The listing builds one solid part. Answer for the finished solid, in the listing's coordinates (mm). A direction names the side the tool comes from. Coordinates: 2 decimals unless noted, no trailing zeros. Order: outer loops, then holes, each group sorted by start corner. A loop starts at its lowest first (then second) coordinate and runs counter-clockwise, first axis right, second up. Notation, with made-up numbers: (9, 36) -> (33, 36) arc R19 ccw to (33, 49) -> close; hole circle Ø11 at (-10.75, 80). An arc over 180 degrees is marked (long way). Put each result on its own line as item: value. Start each with the question number.
```python
from build123d import *

# Parameters (mm, degrees)
SKETCH3_W               = 44.4
SKETCH3_H               = 44.4
BOSS_EXTRUDE1_DEPTH     = 9.7
SKETCH4_W               = 10.3
SKETCH4_H               = 10.3
CUT_EXTRUDE1_DEPTH      = 5.3
SKETCH5_R               = 6
CUT_EXTRUDE2_DEPTH      = 14.3
BOSS_EXTRUDE2_DEPTH     = 5
CUT_EXTRUDE3_DEPTH      = 35.870626966
CUT_EXTRUDE3_DEPTH_BACK = 35.870626966
SKETCH7_R               = 1.5


with BuildPart() as part:
    # Sketch2 → Revolve1 (revolve)
    with BuildSketch(Plane.XY, mode=Mode.PRIVATE) as revolve1_sk:
        with BuildLine():
            Line((-10, 0), (-12, 0))
            ThreePointArc((-12, 0), (-8.485281374, 8.485281374), (0, 12))
            Line((0, 12), (0, 17))
            ThreePointArc((0, 17), (-12.02081528, 12.02081528), (-17, 0))
            Line((-17, 0), (-17, -3.175))
            Line((-17, -3.175), (-10, -3.175))
            Line((-10, -3.175), (-10, 0))
        make_face()
    revolve(revolve1_sk.sketch.rotate(Axis((0, 12, 0), (0, 1, 0)), 180), axis=Axis((0, 12, 0), (0, 1, 0)))

    # Sketch3 → Boss-Extrude1 (add)
    with BuildSketch(Plane.XZ.offset(3.175)):
        Rectangle(SKETCH3_W, SKETCH3_H)
    extrude(amount=BOSS_EXTRUDE1_DEPTH)

    # Sketch4 → Cut-Extrude1 (cut)
    with BuildSketch(Plane.XZ.offset(12.875)):
        with Locations((17.05, -17.05)):
            Rectangle(SKETCH4_W, SKETCH4_H)
    extrude(amount=-CUT_EXTRUDE1_DEPTH, mode=Mode.SUBTRACT)

    # Sketch5 → Cut-Extrude2 (cut)
    with BuildSketch(Plane.XZ.offset(12.875)):
        Circle(SKETCH5_R)
    extrude(amount=-CUT_EXTRUDE2_DEPTH, mode=Mode.SUBTRACT)

    # Sketch6 → Boss-Extrude2 (add)
    with BuildSketch(Plane(origin=(0, -3.175, 0), x_dir=(1, 0, 0), z_dir=(0, 1, 0))):
        with BuildLine():
            Line((-22.2, -22.2), (-22.2, 12.2))
            Line((-22.2, 12.2), (-11.83, 12.2))
            ThreePointArc((-11.83, 12.2), (-11.83, -11.83), (12.2, -11.83))
            Line((12.2, -11.83), (12.2, -22.2))
            Line((12.2, -22.2), (-22.2, -22.2))
        make_face()
    extrude(amount=BOSS_EXTRUDE2_DEPTH)

    # Sketch7 → Cut-Extrude3 (cut, two sides: drawn at the far end of the back side and taken through both)
    with BuildSketch(Plane(origin=(0, 1.825, 0), x_dir=(1, 0, 0), z_dir=(0, 1, 0)).offset(-CUT_EXTRUDE3_DEPTH_BACK)):
        with Locations(Location((-17.5, -17.5, 0), (0, 0, 180))):
            Circle(SKETCH7_R)
        with Locations(Location((17.5, -17.5, 0), (0, 0, 180))):
            Circle(SKETCH7_R)
        with Locations(Location((17.5, 17.5, 0), (0, 0, 180))):
            Circle(SKETCH7_R)
        with Locations(Location((-17.5, 17.5, 0), (0, 0, 180))):
            Circle(SKETCH7_R)
    extrude(amount=CUT_EXTRUDE3_DEPTH + CUT_EXTRUDE3_DEPTH_BACK, mode=Mode.SUBTRACT)


solid = part.part
```
(1) Find the intervals of material crossed by L1, parallel to Z at x = -17.5, y = -7.25; L2, parallel to Z at x = -17, y = -4, in increasing order.
(2) For a pull along Z with two mould halves and no side action, classify faces 4 (the cylindrical face through (-16, -8.09, -17.43)), 5 (the flat face through (-22.2, -6, 0)), 6 (the flat face through (5, 0, -9)), 7 (the cylindrical face through (12.28, -1.61, -11.756)) as released by +Z, released by -Z, zero draft, split by the parting line, or undercut.
(3) The part is cut by section B-B on y = -9.25. Determine the outline of the cut face in (x, z).
(4) Each of these flat-tipped pins is pushed along its axis until it touches: P1, Ø3, axis at x = 16.5, z = -18, coming from the -Y side (3 decimals); P2, Ø1.5, axis at x = -14.5, y = -1, coming from the -Z side; P3, Ø1.6, axis at x = 19.5, y = -11.5, coming from the -Z side. Where does it stop, or does it pass through?
(5) A tool of negligible diameter and unlimited length cuts with its end or side. For faces 1 (the flat face through (17, -10, -11.9)), 2 (the cylindrical face through (-6, -8, 0)), 3 (the cylindrical face through (-10, -2, 0)), from which of +Z, -Z, +X, -X, +Y, -Y can it reach the whole face along a straight path? Write none if from no direction.
(6) The part is cut by section A-A on x = -17.5. Determine the outline of the cut face in (y, z) (3 decimals), plus the area to 3 significant figures.
(7) The part is cut by section D-D on x = 0. Determine the outline of the cut face in (y, z) (3 decimals).
(8) The part is cut by section C-C on z = 17.5. Determine the outline of the cut face in (x, y) (3 decimals), plus the area to 3 significant figures.
Worked out:
1. L1: -22.2 to -19, -16 to 16, 19 to 22.2
1. L2: -22.2 to -18.91, -16.09 to 16.09, 18.91 to 22.2
2. face 4: undercut
2. face 5: zero draft
2. face 6: undercut
2. face 7: split by the parting line
3. outline: (-22.2, -22.2) -> (11.9, -22.2) -> (11.9, -11.9) -> (22.2, -11.9) -> (22.2, 22.2) -> (-22.2, 22.2) -> close; hole circle Ø3 at (-17.5, -17.5); hole circle Ø3 at (-17.5, 17.5); hole circle Ø12 at (0, 0); hole circle Ø3 at (17.5, 17.5)
4. P1: y = -7.575
4. P2: z = -12.2
4. P3: z = -11.9
5. face 1: -Z, +X, -Y
5. face 2: -Y
5. face 3: none
6. outline: (-12.875, -22.2) -> (-3.175, -22.2) -> (-3.175, -19) -> (-12.875, -19) -> close; (-12.875, -16) -> (-3.175, -16) -> (-3.175, -12.2) -> (1.825, -12.2) -> (1.825, 16) -> (-12.875, 16) -> close; (-12.875, 19) -> (1.825, 19) -> (1.825, 22.2) -> (-12.875, 22.2) -> close
6. area: 529 mm2
7. outline: (-12.875, -22.2) -> (-3.175, -22.2) -> (-3.175, -17) -> (0, -17) arc R17 ccw to (1.825, 16.902) -> (1.825, 22.2) -> (-12.875, 22.2) -> (-12.875, 6) -> (-3.175, 6) -> (-3.175, 10) -> (0, 10) -> (0, 12) arc R12 cw to (0, -12) -> (0, -10) -> (-3.175, -10) -> (-3.175, -6) -> (-12.875, -6) -> close
8. outline: (-22.2, -12.875) -> (-19, -12.875) -> (-19, 1.825) -> (-22.2, 1.825) -> close; (-16, -12.875) -> (16, -12.875) -> (16, -3.175) -> (12.2, -3.175) -> (12.2, 1.825) -> (-16, 1.825) -> close; (19, -12.875) -> (22.2, -12.875) -> (22.2, -3.175) -> (19, -3.175) -> close
8. area: 529 mm2
